from build123d import *

# Parameters (mm, degrees)
SKETCH1_W           = 80
SKETCH1_H           = 30.74
SKETCH1_R           = 3
SKETCH1_R_2         = 1.6
BOSS_EXTRUDE1_DEPTH = 3
SKETCH2_R           = 2.1
CUT_EXTRUDE1_DEPTH  = 10
FILLET1_R           = 2


with BuildPart() as part:
    # Sketch1 → Boss-Extrude1 (new body)
    with BuildSketch(Plane(origin=(0, 0, 0), x_dir=(1, 0, 0), z_dir=(0, 1, 0))):
        with Locations((0, 3.63)):
            Rectangle(SKETCH1_W, SKETCH1_H)
        Circle(SKETCH1_R, mode=Mode.SUBTRACT)
        with Locations((0, 7)):
            Circle(SKETCH1_R_2, mode=Mode.SUBTRACT)
        with Locations((-7, 0)):
            Circle(SKETCH1_R_2, mode=Mode.SUBTRACT)
        with Locations((0, -7)):
            Circle(SKETCH1_R_2, mode=Mode.SUBTRACT)
        with Locations((7, 0)):
            Circle(SKETCH1_R_2, mode=Mode.SUBTRACT)
    extrude(amount=-BOSS_EXTRUDE1_DEPTH)

    # Sketch2 → Cut-Extrude1 (cut)
    with BuildSketch(Plane(origin=(0, 0, 0), x_dir=(1, 0, 0), z_dir=(0, 1, 0))):
        with Locations((31.999, 3.93)):
            Circle(SKETCH2_R)
        with Locations((-31.999, 3.93)):
            Circle(SKETCH2_R)
    extrude(amount=-CUT_EXTRUDE1_DEPTH, mode=Mode.SUBTRACT)

    # Fillet1
    fillet1_edges = [part.edges().sort_by_distance(p)[0] for p in [
        (40, -1.5, 11.74),
        (-40, -1.5, 11.74),
    ]]
    fillet(fillet1_edges, radius=FILLET1_R)


solid = part.part
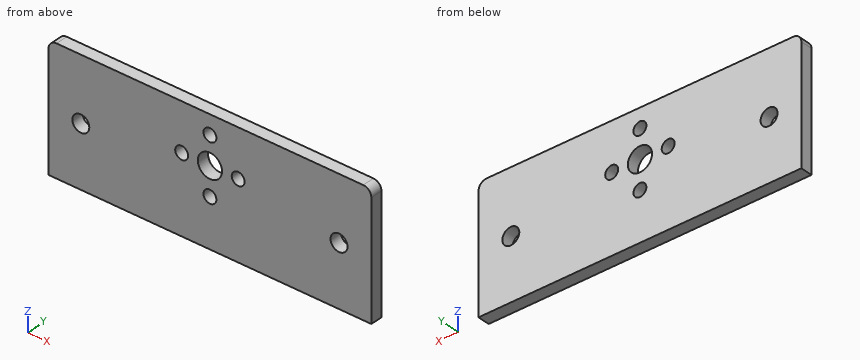
Design review of the part built by this model. Coordinates are the model's own, in mm. Coordinates: 2 decimals unless noted, no trailing zeros. Loops run counter-clockwise (first coordinate to the right, second up) from the corner with the lowest first, then second, coordinate; pieces in that order, holes last. Notation, with made-up numbers: (69.25, 15) - (85.25, 15) arc R18 cw to (85.25, 39) - close; hole circle Ø10 at (65.25, -17.75). An arc over 180 degrees is marked (long way). Use CSV: the item, a comma, the result in double quotes. Start each with the question number.
1. Add section B-B on y = -2.2. Give the boundary of the cut face in (x, z).
2. Add section D-D on x = 0. Give the boundary of the cut face in (y, z).
3. Add section A-A on z = 7. Give the boundary of the cut face in (x, y).
4. Add section C-C on z = -3.93. Give the boundary of the cut face in (x, y), plus the area to 3 significant figures.
5. To check wall thickness, follow probe 1 along X at (y, z) = (-1.9, 0); probe 2 along Z at (x, y) = (0, -0.7); probe 3 along X at (y, z) = (-1.3, -3.93). State the ranges of each line that lie inside material, in increasing order.
Resolved:
1,outline,"(-40, -19) - (40, -19) - (40, 9.74) arc R2 ccw to (38, 11.74) - (-38, 11.74) arc R2 ccw to (-40, 9.74) - close; hole circle Ø4.2 at (-32, -3.93); hole circle Ø3.2 at (-7, 0); hole circle Ø6 at (0, 0); hole circle Ø3.2 at (0, -7); hole circle Ø3.2 at (0, 7); hole circle Ø3.2 at (7, 0); hole circle Ø4.2 at (32, -3.93)"
2,outline,"(-3, -19) - (0, -19) - (0, -8.6) - (-3, -8.6) - close; (-3, -5.4) - (0, -5.4) - (0, -3) - (-3, -3) - close; (-3, 3) - (0, 3) - (0, 5.4) - (-3, 5.4) - close; (-3, 8.6) - (0, 8.6) - (0, 11.74) - (-3, 11.74) - close"
3,outline,"(-40, -3) - (-1.6, -3) - (-1.6, 0) - (-40, 0) - close; (1.6, -3) - (40, -3) - (40, 0) - (1.6, 0) - close"
4,outline,"(-40, -3) - (-34.1, -3) - (-34.1, 0) - (-40, 0) - close; (-29.9, -3) - (29.9, -3) - (29.9, 0) - (-29.9, 0) - close; (34.1, -3) - (40, -3) - (40, 0) - (34.1, 0) - close"
4,area,"215 mm2"
5,probe 1,"-40 to -8.6, -5.4 to -3, 3 to 5.4, 8.6 to 40"
5,probe 2,"-19 to -8.6, -5.4 to -3, 3 to 5.4, 8.6 to 11.74"
5,probe 3,"-40 to -34.1, -29.9 to 29.9, 34.1 to 40"
